Autodesk Inventor part; units mm, degrees
ref_plane "YZ Plane" through (0, 0, 0) normal (1, 0, 0) x (0, 1, 0)
ref_plane "XZ Plane" through (0, 0, 0) normal (0, 1, 0) x (-1, 0, 0)
ref_plane "XY Plane" through (0, 0, 0) normal (0, 0, 1) x (1, 0, 0)
sketch "Sketch1" plane through (0, 0, 0) normal (1, 0, 0) x (0, 1, 0)
  line L0 (130.7193, 523.9242) -> (675.7193, 523.9242)
  line L1 (675.7193, 523.9242) -> (675.7193, -1051.0758)
  line L2 (675.7193, -1051.0758) -> (130.7193, -1051.0758)
  line L3 (130.7193, -1051.0758) -> (130.7193, 523.9242)
  line L4 (213.2193, -931.0758) -> (593.2193, -931.0758)
  line L5 (593.2193, -931.0758) -> (593.2193, 168.9242)
  line L6 (593.2193, 168.9242) -> (213.2193, 168.9242)
  line L7 (213.2193, 168.9242) -> (213.2193, -931.0758)
  point P0 (0, 0)
  dimension "b" = 545
  dimension "d1" = 1575
  dimension "d4" = 380
  dimension "d5" = 82.5
  dimension "d6" = 1100
  dimension "d8" = 120
extrude "Extrusion1" add sketch "Sketch1" along normal blind 12 contours L0 L1 L2 L3 | L7 L6 L5 L4
extrude "Extrusion2" cut sketch "Sketch1" along normal up to next contours L7 L6 L5 L4
equation "\"d5\" = -0.5 * d4 + 0.5 * b"
properties part number "CUT PART G-01" material "Wood (Birch)"
For this review, take the finished solid that the model builds, in its own axes (mm). Coordinates: 2 decimals unless noted, no trailing zeros. Write each loop counter-clockwise with the first axis right and the second up, starting at its lowest first coordinate (ties: lowest second). Pieces come first, ordered by that corner, then holes. Notation, with made-up numbers: (45.25, 0) - (84.25, 0) arc R24 ccw to (84.25, 31) - close; hole circle Ø5 at (73.5, -34.75). An arc over 180 degrees is marked (long way). Put each result on its own line as item: value.
1. Wall thickness on probe 1 along Z at (x, y) = (6, 314); probe 2 along Y at (x, z) = (3.75, -182): over which ranges is each line inside the solid? List them lowest first.
Values found:
probe 1: -1051.08 to -931.08, 168.92 to 523.92
probe 2: 130.72 to 213.22, 593.22 to 675.72
2. Add section B-B, the plane y = 544. Give the boundary of the cut face in (x, z), then the cut area to 3 significant figures.
Values found:
outline: (0, -1051.08) - (12, -1051.08) - (12, -931.08) - (0, -931.08) - close; (0, 168.92) - (12, 168.92) - (12, 523.92) - (0, 523.92) - close
area: 5,700 mm²
3. Add section C-C, the plane x = 5. Give the boundary of the cut face in (y, z).
Values found:
outline: (130.72, -1051.08) - (675.72, -1051.08) - (675.72, 523.92) - (130.72, 523.92) - close; hole (213.22, -931.08) - (593.22, -931.08) - (593.22, 168.92) - (213.22, 168.92) - close
4. Add section A-A, the plane z = -350. Give the boundary of the cut face in (x, y), then the cut area to 3 significant figures.
Values found:
outline: (0, 130.72) - (12, 130.72) - (12, 213.22) - (0, 213.22) - close; (0, 593.22) - (12, 593.22) - (12, 675.72) - (0, 675.72) - close
area: 1,980 mm²
